Read the model definition and answer for the solid it produces. Units are mm, in the model's axes. Face numbers are marked on the shaded views. A direction names the side the tool comes from. Give positions to 0.01 mm unless a question says otherwise; leave off trailing zeros. Order: outer loops, then holes, each group sorted by start corner. A loop starts at its lowest first (then second) coordinate and runs counter-clockwise, first axis right, second up. Notation, with made-up numbers: (83.25, 28) - (129.25, 28) arc R15 ccw to (129.25, 50) - close; hole circle Ø11 at (-20, -34.75). An arc over 180 degrees is marked (long way). Write each question's results on one line, items separated by ' | '. Start each with the question number.
Q1. Find section C-C on z = -44. Give the vertices of the cut face in (x, y).
Q2. For a pull along X with two mould halves and no side action, classify the marked faces 5, 6, 7 and 8 as +X half, -X half, draft (parallel to the pull), parting line (faces both ways), or undercut.
Q3. Find section B-B on x = 0. Give the vertices of the cut face in (y, z), and give its area (4 significant figures).
Q4. Find section D-D on y = 60. Give the vertices of the cut face in (x, z), and give its area (3 significant figures).
Q5. A tool of negligible diameter and unlimited length cuts with its end or side. For the marked faces 1, 2, 3 and 4, from which of +Z, -Z, +X, -X, +Y, -Y can it reach the whole face along a straight path? Write none if from no direction.
Q6. Flat-ended cylindrical pins translate along their axes: P1, Ø5, axis at y = 11, z = 0, coming from the +X side; P2, Ø10, axis at x = -55, z = 8, coming from the +Y side; P3, Ø2.5, axis at y = 147, z = -1.5, coming from the -X side; P4, Ø5, axis at x = -39, z = -22, coming from the +Y side. Find the tip coordinate at first contact, or state that the pin passes through.
Q7. Find section A-A on y = 11. Give the vertices of the cut face in (x, z).
Q8. Find the intervals of material crossed by line 1 along Y through (x, z) = (-67, -44); line 2 along Y through (x, z) = (-66, 0); line 3 along X through (y, z) = (41, -47.5), in increasing order. Write a range as from..to.
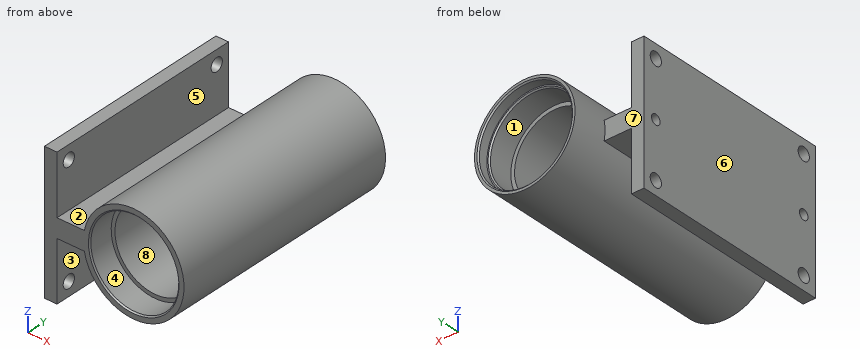
from build123d import *

# Parameters (mm, degrees)
SCHIZZO1_R        = 32
ESTRUSIONE1_DEPTH = 160
SCHIZZO2_R        = 40
SCHIZZO2_R_2      = 35
ESTRUSIONE2_DEPTH = 20
SCHIZZO4_R        = 5.25
ESTRUSIONE4_DEPTH = 20
SCHIZZO5_R        = 4
ESTRUSIONE5_DEPTH = 12
SCHIZZO6_R        = 40
SCHIZZO6_R_2      = 37
ESTRUSIONE6_DEPTH = 8
SCHIZZO7_R        = 35
ESTRUSIONE7_DEPTH = 20
SMUSSO1_SIZE      = 1


with BuildPart() as part:
    # Schizzo1 → Estrusione1 (new body)
    with BuildSketch(Plane(origin=(0, 0, 0), x_dir=(1, 0, 0), z_dir=(0, 1, 0))):
        with BuildLine():
            Line((-39.290584114, 7.5), (-61, 7.5))
            Line((-61, 7.5), (-61, 55))
            Line((-61, 55), (-71, 55))
            Line((-71, 55), (-71, -55))
            Line((-71, -55), (-61, -55))
            Line((-61, -55), (-61, -7.5))
            Line((-61, -7.5), (-39.290584114, -7.5))
            ThreePointArc((-39.290584114, -7.5), (40, 0), (-39.290584114, 7.5))
        make_face()
        with Locations(Location((0, 0, 0), (0, 0, 270))):
            Circle(SCHIZZO1_R, mode=Mode.SUBTRACT)
    extrude(amount=ESTRUSIONE1_DEPTH)

    # Schizzo2 → Estrusione2 (add)
    with BuildSketch(Plane(origin=(0, 160, 0), x_dir=(1, 0, 0), z_dir=(0, 1, 0))):
        with Locations(Location((0, 0, 0), (0, 0, 169.193077125))):
            Circle(SCHIZZO2_R)
        with Locations(Location((0, 0, 0), (0, 0, 270))):
            Circle(SCHIZZO2_R_2, mode=Mode.SUBTRACT)
    extrude(amount=ESTRUSIONE2_DEPTH)

    # Schizzo4 → Estrusione4 (cut)
    with BuildSketch(Plane.ZY.offset(71)):
        with Locations((-44, 149)):
            Circle(SCHIZZO4_R)
        with Locations((44, 149)):
            Circle(SCHIZZO4_R)
        with Locations((44, 11)):
            Circle(SCHIZZO4_R)
        with Locations((-44, 11)):
            Circle(SCHIZZO4_R)
    extrude(amount=-ESTRUSIONE4_DEPTH, mode=Mode.SUBTRACT)

    # Schizzo5 → Estrusione5 (cut)
    with BuildSketch(Plane.ZY.offset(71)):
        with Locations((0, 149)):
            Circle(SCHIZZO5_R)
        with Locations(Location((0, 11, 0), (0, 0, 180))):
            Circle(SCHIZZO5_R)
    extrude(amount=-ESTRUSIONE5_DEPTH, mode=Mode.SUBTRACT)

    # Schizzo6 → Estrusione6 (add)
    with BuildSketch(Plane(origin=(0, 180, 0), x_dir=(1, 0, 0), z_dir=(0, 1, 0))):
        with Locations(Location((0, 0, 0), (0, 0, 169.193077125))):
            Circle(SCHIZZO6_R)
        with Locations(Location((0, 0, 0), (0, 0, 270))):
            Circle(SCHIZZO6_R_2, mode=Mode.SUBTRACT)
    extrude(amount=ESTRUSIONE6_DEPTH)

    # Schizzo7 → Estrusione7 (cut)
    with BuildSketch(Plane.XZ):
        with Locations(Location((0, 0, 0), (0, 0, 90))):
            Circle(SCHIZZO7_R)
    extrude(amount=-ESTRUSIONE7_DEPTH, mode=Mode.SUBTRACT)

    # Smusso1
    smusso1_edges = [part.edges().sort_by_distance(p)[0] for p in [
        (0, 180, -35),
        (0, 188, -37),
        (0, 0, -35),
    ]]
    chamfer(smusso1_edges, length=SMUSSO1_SIZE)


solid = part.part
Working result:
1) outline: (-71, 0) - (-61, 0) - (-61, 5.75) - (-71, 5.75) - close; (-71, 16.25) - (-61, 16.25) - (-61, 143.75) - (-71, 143.75) - close; (-71, 154.25) - (-61, 154.25) - (-61, 160) - (-71, 160) - close
2) face 5: undercut | face 6: -X half | face 7: draft | face 8: undercut
3) outline: (0, -40) - (188, -40) - (188, -38) - (187, -37) - (180, -37) - (180, -36) - (179, -35) - (160, -35) - (160, -32) - (20, -32) - (20, -35) - (1, -35) - (0, -36) - close; (0, 36) - (1, 35) - (20, 35) - (20, 32) - (160, 32) - (160, 35) - (179, 35) - (180, 36) - (180, 37) - (187, 37) - (188, 38) - (188, 40) - (0, 40) - close | area: 2,685 mm²
4) outline: (-71, -55) - (-61, -55) - (-61, -7.5) - (-39.29, -7.5) arc R40 ccw (long way) to (-39.29, 7.5) - (-61, 7.5) - (-61, 55) - (-71, 55) - close; hole circle Ø64 at (0, 0) | area: 3,230 mm²
5) face 1: +Y | face 2: +Z, +Y, -Y | face 3: -Z, +Y, -Y | face 4: -Y
6) P1: x = 40 | P2: y = 160 | P3: x = -59 | P4: through
7) outline: (-71, -55) - (-61, -55) - (-61, -49.25) - (-71, -49.25) - close; (-71, -38.75) - (-61, -38.75) - (-61, -7.5) - (-39.29, -7.5) arc R40 ccw (long way) to (-39.29, 7.5) - (-61, 7.5) - (-61, 38.75) - (-71, 38.75) - (-71, 4) - (-59, 4) - (-59, -4) - (-71, -4) - close; (-71, 49.25) - (-61, 49.25) - (-61, 55) - (-71, 55) - close; hole circle Ø70 at (0, 0)
8) line 1: 0..5.75, 16.25..143.75, 154.25..160 | line 2: 0..7, 15..145, 153..160 | line 3: -71..-61
